```python
from build123d import *

# Parameters (mm, degrees)
F0_W     = 152.4
F0_H     = 241.3
F0_R     = 7.14375
F1_DEPTH = 12.7
F3_W     = 139.7
F3_H     = 203.2
F4_DEPTH = 12.7
F7_DEPTH = 12.7


with BuildPart() as f1:
    # F0 (on Top) → F1 (new body)
    with BuildSketch(Plane.XY):
        Rectangle(F0_W, F0_H)
        with Locations((-50.8, -63.5)):
            Circle(F0_R, mode=Mode.SUBTRACT)
        with Locations((50.8, -63.5)):
            Circle(F0_R, mode=Mode.SUBTRACT)
        with Locations((-50.8, 63.5)):
            Circle(F0_R, mode=Mode.SUBTRACT)
        with Locations((50.8, 63.5)):
            Circle(F0_R, mode=Mode.SUBTRACT)
    extrude(amount=F1_DEPTH)



with BuildPart() as f4:
    # F3 (on offset) → F4 (new body)
    with BuildSketch(Plane.XY.offset(222.25)):
        with Locations((-38.1, 0)):
            Rectangle(F3_W, F3_H)
        with BuildLine():
            ThreePointArc((-83.312, -69.088), (-88.9, -63.5), (-83.312, -57.912))
            Line((-83.312, -57.912), (-69.088, -57.912))
            ThreePointArc((-69.088, -57.912), (-63.5, -63.5), (-69.088, -69.088))
            Line((-69.088, -69.088), (-83.312, -69.088))
        make_face(mode=Mode.SUBTRACT)
        with BuildLine():
            ThreePointArc((-4.5457187648, -69.088), (-10.1337187648, -63.5), (-4.5457187648, -57.912))
            Line((-4.5457187648, -57.912), (9.6782812352, -57.912))
            ThreePointArc((9.6782812352, -57.912), (15.2662812352, -63.5), (9.6782812352, -69.088))
            Line((9.6782812352, -69.088), (-4.5457187648, -69.088))
        make_face(mode=Mode.SUBTRACT)
        with BuildLine():
            Line((-69.088, 57.912), (-83.312, 57.912))
            ThreePointArc((-83.312, 57.912), (-88.9, 63.5), (-83.312, 69.088))
            Line((-83.312, 69.088), (-69.088, 69.088))
            ThreePointArc((-69.088, 69.088), (-63.5, 63.5), (-69.088, 57.912))
        make_face(mode=Mode.SUBTRACT)
        with BuildLine():
            Line((9.6782812352, 57.912), (-4.5457187648, 57.912))
            ThreePointArc((-4.5457187648, 57.912), (-10.1337187648, 63.5), (-4.5457187648, 69.088))
            Line((-4.5457187648, 69.088), (9.6782812352, 69.088))
            ThreePointArc((9.6782812352, 69.088), (15.2662812352, 63.5), (9.6782812352, 57.912))
        make_face(mode=Mode.SUBTRACT)
    extrude(amount=-F4_DEPTH)


with BuildPart() as f1_1:
    add(f1.part)

    add(f4.part)  # F7 merges F4
    # F6 (on offset) → F7 (join)
    with BuildSketch(Plane.XZ.offset(95.25)):
        Polygon((31.75, 209.55), (-107.95, 209.55), (-76.2, 12.7), (76.2, 12.7), align=None)
    extrude(amount=F7_DEPTH)

    # F8: F1 across plane


with BuildPart() as f1_2:
    add(f1_1.part)
    add(f1_1.part.mirror(Plane.XZ))


solid = f1_2.part
```
Verification items for the finished model (mm, model axes). A direction names the side the tool comes from. Give positions to 0.01 mm unless a question says otherwise; leave off trailing zeros. Loops run counter-clockwise (first coordinate to the right, second up) from the corner with the lowest first, then second, coordinate; pieces in that order, holes last. Notation, with made-up numbers: M 76.5,-38.75 L 84.5,-38.75 A11 ccw 84.5,-24.75 Z; hole C -28.75,85 d8. An arc over 180 degrees is marked long. One line per question, with ' | ' between items.
Item 1: Thickness scan on line 1 (X direction, y = -63, z = 3); line 2 (Y direction, x = -50.8, z = 7.25); line 3 (Y direction, x = -69.5, z = 28). Record the ranges inside material, lowest first. Write a range as [from, to].
Completed:
line 1: x = [-76.2, -57.93], [-43.67, 43.67], [57.93, 76.2] | line 2: y = [-120.65, -70.64], [-56.36, 56.36], [70.64, 120.65] | line 3: y = [-107.95, -95.25], [95.25, 107.95]
Item 2: Section check D-D, the plane x = 50.8. Record the cut outline in (y, z).
Completed:
outline: M -120.65,0 L -70.64,0 L -70.64,12.7 L -95.25,12.7 L -95.25,125.19 L -107.95,125.19 L -107.95,12.7 L -120.65,12.7 Z; M -56.36,0 L 56.36,0 L 56.36,12.7 L -56.36,12.7 Z; M 70.64,0 L 120.65,0 L 120.65,12.7 L 107.95,12.7 L 107.95,125.19 L 95.25,125.19 L 95.25,12.7 L 70.64,12.7 Z
Item 3: Section check A-A, the plane y = -30. Record the cut outline in (x, z), plus the area to 3 significant figures.
Completed:
outline: M -107.95,209.55 L 31.75,209.55 L 31.75,222.25 L -107.95,222.25 Z; M -76.2,0 L 76.2,0 L 76.2,12.7 L -76.2,12.7 Z | area: 3,710 mm^2
Item 4: Section check B-B, the plane z = 88. Record the cut outline in (x, y), plus the area to 3 significant figures.
Completed:
outline: M -88.35,-107.95 L 59.2,-107.95 L 59.2,-95.25 L -88.35,-95.25 Z; M -88.35,95.25 L 59.2,95.25 L 59.2,107.95 L -88.35,107.95 Z | area: 3,750 mm^2
Item 5: Depth check by flat-ended pin: P1, Ø10, axis at x = -43.5, z = 217, coming from the +Y side; P2, Ø6.5, axis at y = -16.5, z = 219, coming from the +X side; P3, Ø14, axis at x = 21, y = 114.5, coming from the +Z side. Enter the tip coordinate at first touch or a pass-through.
Completed:
P1: stops at y = 101.6 | P2: stops at x = 31.75 | P3: stops at z = 209.55
Item 6: Draft check along X on faces 1 (the face through (-76.2, -2, 6)), 2 (the face through (-76, 69.088, 216)), 3 (the face through (-10.132, -63.623, 215.989)), 4 (the face through (-1, -120.65, 6)). Enter one of: +X half, -X half, draft (parallel to the pull), parting line (faces both ways), or undercut.
Completed:
face 1: -X half | face 2: undercut | face 3: undercut | face 4: draft
Item 7: Tool access check on faces 5 (the face through (-39, -101.6, 216)), 6 (the face through (-39, 101.6, 216)), 7 (the face through (15.265, 63.623, 215.989)). Record the directions out of +Z, -Z, +X, -X, +Y, -Y that give a thin tool (end or side, any length) a straight path to the whole face; none if there is none.
Completed:
face 5: +Z, +X, -X, -Y | face 6: +Z, +X, -X, +Y | face 7: +Z
Item 8: Section check C-C, the plane y = -63.5. Record the cut outline in (x, z), plus the area to 3 significant figures.
Completed:
outline: M -107.95,209.55 L -88.9,209.55 L -88.9,222.25 L -107.95,222.25 Z; M -76.2,0 L -57.94,0 L -57.94,12.7 L -76.2,12.7 Z; M -63.5,209.55 L -10.13,209.55 L -10.13,222.25 L -63.5,222.25 Z; M -43.66,0 L 43.66,0 L 43.66,12.7 L -43.66,12.7 Z; M 15.27,209.55 L 31.75,209.55 L 31.75,222.25 L 15.27,222.25 Z; M 57.94,0 L 76.2,0 L 76.2,12.7 L 57.94,12.7 Z | area: 2,700 mm^2
